Part model, mm, in its own coordinate system. A direction names the side the tool comes from. Round coordinates to 2 decimals unless told otherwise and drop trailing zeros. Loops run counter-clockwise (first coordinate to the right, second up) from the corner with the lowest first, then second, coordinate; pieces in that order, holes last. Notation, with made-up numbers: (-19, 38) - (-13, 38) arc R14 cw to (-13, 47) - close; hole circle Ø7 at (81, 1). An arc over 180 degrees is marked (long way). Write each question's results on one line, items separated by ' | '. Start each with the question number.
(1) Mould opens along Z. For faces 3 (the face through (-8.79, -0.867, 100.407)), 4 (the face through (-9.921, -1, 50)), 5 (the face through (0.87, 19.98, 49.69)), 6 (the face through (0.867, 19.4, 98.404)) say: released by +Z, released by -Z, zero draft, split by the parting line, or undercut.
(2) Cut at D-D, the plane y = 3. List the corners of the cut face in (x, z), then the cut area to 3 significant figures.
(3) Flat gauge pins, fed straight in: P1, Ø3, axis at y = 9, z = 52, coming from the -X side; P2, Ø3, axis at y = 19.725, z = 5.675, coming from the -X side; P3, Ø6.5, axis at x = -7.5, z = 34, coming from the +Y side. Where does each tip first touch, or does it go through?
(4) Cut at A-A, the plane z = 50.8. List the corners of the cut face in (x, y), then the cut area to 3 significant figures.
(5) Drill centre lines: L1, parallel to Y at x = -3.5, z = 58; L2, parallel to X at y = 12.5, z = 77; L3, parallel to Z at x = 1, y = 19.75. Where is each one in solid material? Low to high.
(6) Cut at C-C, the plane z = 7. List the corners of the cut face in (x, y) (3 decimals).
(7) Cut at B-B, the plane z = 73.5. List the corners of the cut face in (x, y).
(8) Tool access for faces 1 (the face through (-6, 0, 50)), 2 (the face through (1.709, 14, 50)): list every direction of +Z, -Z, +X, -X, +Y, -Y with a clear straight run to the whole face (end or side of a thin tool).
from build123d import *

# Parameters (mm, degrees)
F1_DEPTH = 101.6
F2_R     = 3.69316
F3_R     = 1.98374
F4_R     = 1.8288
F4_R_2   = 2.5
F5_DEPTH = 1.70942
F6_R     = 5.674995
F7_R     = 3.96875
F8_R     = 1.8288
F9_DEPTH = 1.70942


with BuildPart() as f1:
    # F0 (on Top) → F1 (new body)
    with BuildSketch(Plane.XY):
        Polygon((0, 25.4), (0, 0), (-9.92124, 0), (-9.92124, -1.70942), (1.70942, -1.70942), (1.70942, 25.4), align=None)
    extrude(amount=F1_DEPTH)

    # F2
    f2_edges = [f1.edges().sort_by_distance(p)[0] for p in [
        (1.70942, -1.70942, 50.8),
    ]]
    fillet(f2_edges, radius=F2_R)

    # F3
    f3_edges = [f1.edges().sort_by_distance(p)[0] for p in [
        (0, 0, 50.8),
    ]]
    fillet(f3_edges, radius=F3_R)

    # F4 (on face) → F5 (cut, through all)
    with BuildSketch(Plane.YZ.offset(1.70942)):
        with Locations((21.43125, 50.8)):
            Circle(F4_R)
        with Locations((5.95249, 50.8)):
            Circle(F4_R)
        with Locations((19.725, 95.925)):
            Circle(F4_R_2)
        with Locations((19.725, 5.675)):
            Circle(F4_R_2)
    extrude(amount=-F5_DEPTH, mode=Mode.SUBTRACT)

    # F6
    f6_edges = [f1.edges().sort_by_distance(p)[0] for p in [
        (0.85471, 25.4, 101.6),
        (0.85471, 25.4, 0),
    ]]
    fillet(f6_edges, radius=F6_R)

    # F7
    f7_edges = [f1.edges().sort_by_distance(p)[0] for p in [
        (-9.92124, -0.85471, 0),
        (-9.92124, -0.85471, 101.6),
    ]]
    fillet(f7_edges, radius=F7_R)

    # F8 (on face) → F9 (cut, through all)
    with BuildSketch(Plane.XZ.offset(1.70942)):
        with Locations((-5.95249, 97.63125)):
            Circle(F8_R)
        with Locations((-5.95249, 3.96875)):
            Circle(F8_R)
    extrude(amount=-F9_DEPTH, mode=Mode.SUBTRACT)


solid = f1.part
A:
1) face 3: released by +Z | face 4: zero draft | face 5: undercut | face 6: undercut
2) outline: (0, 0) - (1.71, 0) - (1.71, 101.6) - (0, 101.6) - close | area: 174 mm2
3) P1: x = 0 | P2: through | P3: y = 0
4) outline: (-9.92, -1.71) - (-1.98, -1.71) arc R3.69 ccw to (1.71, 1.98) - (1.71, 4.12) - (0, 4.12) - (0, 1.98) arc R1.98 cw to (-1.98, 0) - (-9.92, 0) - close; (0, 7.78) - (1.71, 7.78) - (1.71, 19.6) - (0, 19.6) - close; (0, 23.26) - (1.71, 23.26) - (1.71, 25.4) - (0, 25.4) - close | area: 48.7 mm2
5) L1: -1.71 to 0 | L2: 0 to 1.71 | L3: 0 to 3.18, 8.17 to 50.08, 51.52 to 93.43, 98.42 to 101.6
6) outline: (-9.921, -1.709) - (-1.984, -1.709) arc R3.693 ccw to (1.709, 1.984) - (1.709, 17.605) - (0, 17.605) - (0, 1.984) arc R1.984 cw to (-1.984, 0) - (-9.921, 0) - close; (0, 21.845) - (1.709, 21.845) - (1.709, 25.4) - (0, 25.4) - close
7) outline: (-9.92, -1.71) - (-1.98, -1.71) arc R3.69 ccw to (1.71, 1.98) - (1.71, 25.4) - (0, 25.4) - (0, 1.98) arc R1.98 cw to (-1.98, 0) - (-9.92, 0) - close
8) face 1: +Z, -Z, -X, +Y | face 2: +Z, -Z, +X, +Y, -Y
